Geometry: see drawing. Coordinates: mm, zero at the bounding-box minimum. A direction names the side the tool comes from. Round coordinates to 2 decimals unless told otherwise and drop trailing zeros. Order: outer loops, then holes, each group sorted by start corner. A loop starts at its lowest first (then second) coordinate and runs counter-clockwise, first axis right, second up. Notation, with made-up numbers: (83.5, 37) -> (98.5, 37) arc R20 ccw to (98.5, 69) -> close; hole circle Ø4 at (87, 62.5). An arc over 180 degrees is marked (long way). One line per item, written item: value. Start each with the question number.
1) Pin query (flat end, axial travel): P1, Ø1, axis at y = 6.5, z = 3.5, coming from the +X side; P2, Ø4, axis at x = 1, y = 7.5, coming from the -Z side; P3, Ø3, axis at x = 4.5, y = 6, coming from the +Z side. Return the tip coordinate at first contact, or that it passes through.
2) Section B-B (y = 0.75). Return the cut outline in (x, z).
3) Reachability of the marked faces 1 and 2 from +Z, -Z, +X, -X, +Y, -Y: full face, straight path, thin tool, end or side. Return the list, or none.
4) Section A-A (x = 4.8). Return the cut outline in (y, z).
5) Ray query, L1, parallel to Y at x = 2, z = 7.75; L2, parallel to Z at x = 4.75, y = 8.75; L3, parallel to X at y = 1.5, z = 7. Return the intervals inside material, ascending.
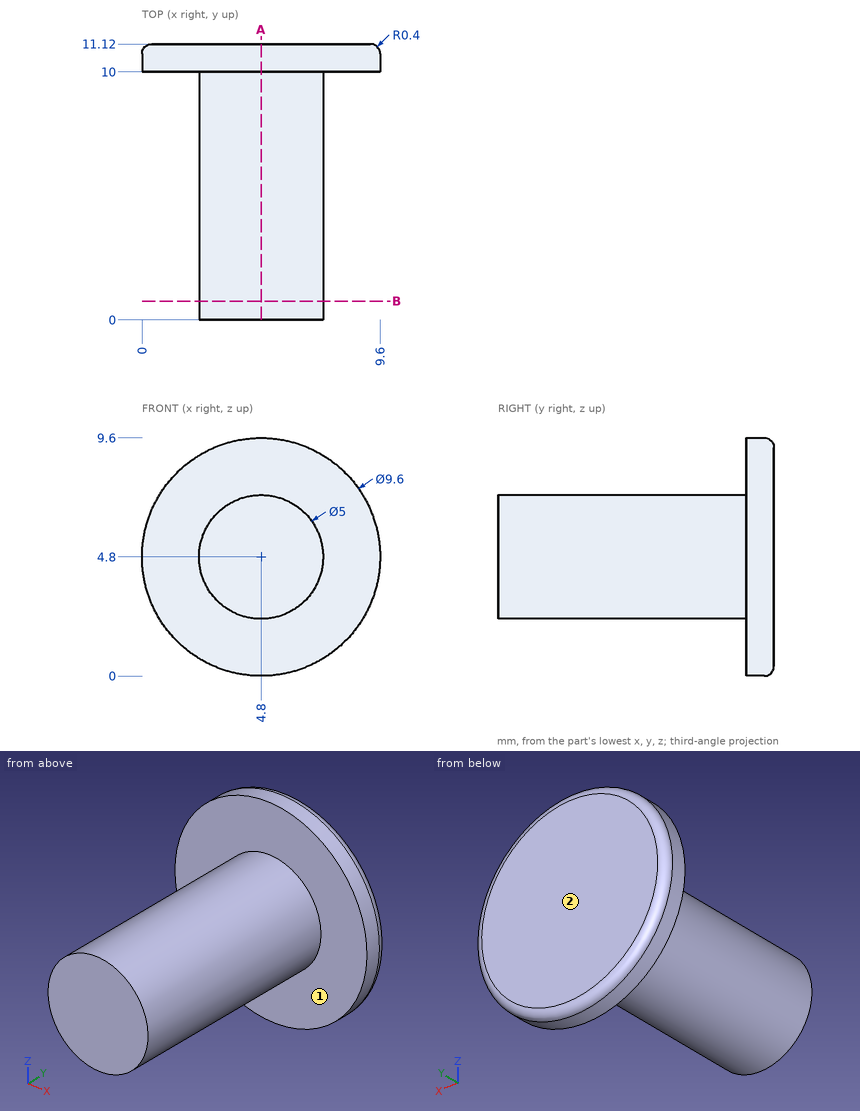
Findings:
1. P1: x = 7.17
1. P2: z = 3.07
1. P3: z = 7.3
2. outline: circle Ø5 at (4.8, 4.8)
3. face 1: -Y
3. face 2: +Z, -Z, +X, -X, +Y
4. outline: (0, 2.3) -> (10, 2.3) -> (10, 0) -> (10.72, 0) arc R0.4 ccw to (11.12, 0.4) -> (11.12, 9.2) arc R0.4 ccw to (10.72, 9.6) -> (10, 9.6) -> (10, 7.3) -> (0, 7.3) -> close
5. L1: 10 to 11.12
5. L2: 2.3 to 7.3
5. L3: 3.61 to 5.99
